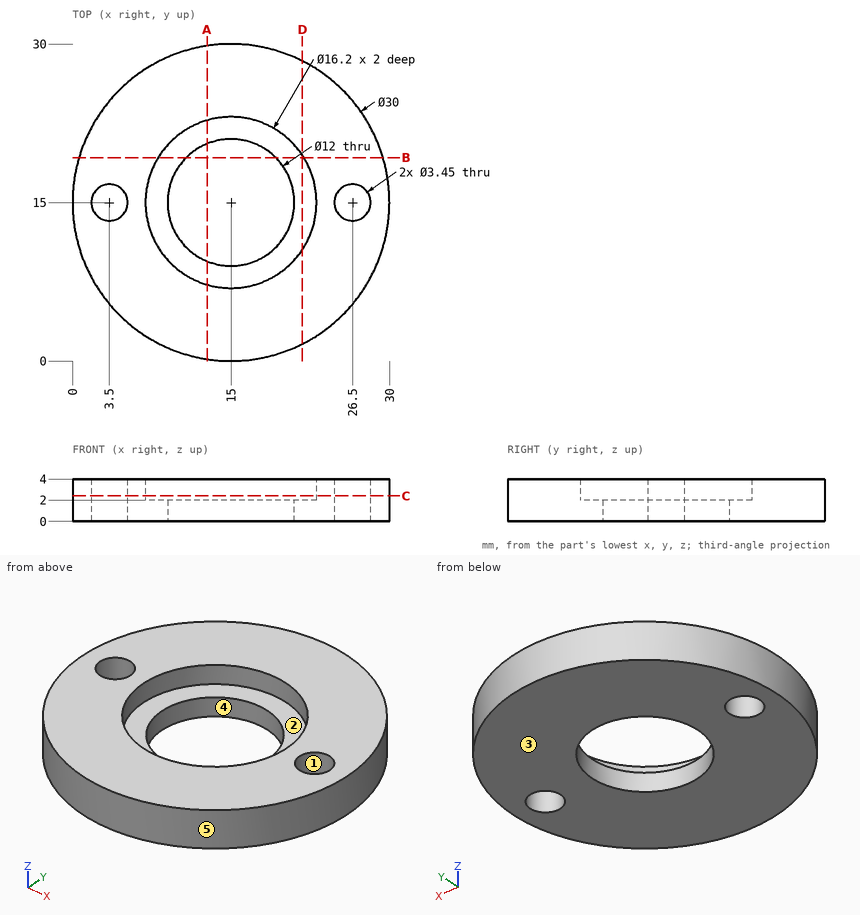
Here's the drawing with two shaded views (mm, measured from the low corner). I have some questions. A direction names the side the tool comes from. Round coordinates to 2 decimals unless told otherwise and drop trailing zeros. Write each loop counter-clockwise with the first axis right and the second up, starting at its lowest first coordinate (ties: lowest second). Pieces come first, ordered by that corner, then holes. Notation, with made-up numbers: M 16,80 L 20,80 A14 ccw 20,103 Z; hole C -39,49.5 d4. An arc over 180 degrees is marked long. Write each question's results on one line, items separated by ' | '. Start each with the question number.
1. Imagine slicing it at A-A on x = 12.75. List the corners of the cut face in (y, z) for me.
2. On a 3-axis mill with a long thin cutter (end or side, diameter ignored), from which of +Z, -Z, +X, -X, +Y, -Y can I reach the whole of each face in a straight line? I mean the marked faces 1 and 2. Say none if no direction works.
3. I need wall thicknesses on L1, parallel to Y at x = 15, z = 1; L2, parallel to X at y = 16.5, z = 2.95; L3, parallel to Y at x = 15, z = 2.6. Which ranges of each line are inside material? Lowest first, please. Write a range as from..to.
4. Imagine slicing it at C-C on z = 2.4. List the corners of the cut face in (x, y) for me (3 decimals), and give its area (3 significant figures).
5. I'm going to push a flat-ended pin straight in: pin 1 Ø9.5 at (x, y) = (15, 15) entering from +Z. Where does the tip first touch, or does it pass through?
6. Imagine slicing it at D-D on x = 21.75. List the corners of the cut face in (y, z) for me, and give its area (3 significant figures).
7. Thinking about a two-plate mould opening in Y: for the marked faces 3, 4 and 5, which applies, +Y half, -Y half, draft (parallel to the pull), parting line (faces both ways), or undercut?
8. Imagine slicing it at B-B on y = 19.25. List the corners of the cut face in (x, z) for me, and give its area (3 significant figures).
Result sheet:
1) outline: M 0.17,0 L 9.44,0 L 9.44,2 L 7.22,2 L 7.22,4 L 0.17,4 Z; M 20.56,0 L 29.83,0 L 29.83,4 L 22.78,4 L 22.78,2 L 20.56,2 Z
2) face 1: +Z, -Z | face 2: +Z
3) L1: y = 0..9, 21..30 | L2: x = 0.08..2.65, 4.35..7.04, 22.96..25.65, 27.35..29.92 | L3: y = 0..6.9, 23.1..30
4) outline: C 15,15 d30; hole C 3.5,15 d3.45; hole C 15,15 d16.2; hole C 26.5,15 d3.45 | area: 482 mm^2
5) pin 1: passes through
6) outline: M 1.6,0 L 28.4,0 L 28.4,4 L 19.48,4 L 19.48,2 L 10.52,2 L 10.52,4 L 1.6,4 Z | area: 89.3 mm^2
7) face 3: draft | face 4: undercut | face 5: parting line
8) outline: M 0.61,0 L 10.76,0 L 10.76,2 L 8.1,2 L 8.1,4 L 0.61,4 Z; M 19.24,0 L 29.39,0 L 29.39,4 L 21.9,4 L 21.9,2 L 19.24,2 Z | area: 70.6 mm^2
